from build123d import *

# Parameters (mm, degrees)
F0_W          = 25.4
F0_H          = 25.4
F1_DEPTH      = 584.2
F2_W          = 25.4
F2_H          = 25.4
F3_DEPTH      = 279.4
F3_DEPTH_BACK = 25.4
F5_DEPTH      = 584.201
F5_DEPTH_BACK = 584.201
F6_W          = 25.4
F6_H          = 25.4
F7_DEPTH      = 279.4
F8_W          = 25.4
F8_H          = 25.4
F9_DEPTH      = 355.6
F10_W         = 25.4
F10_H         = 25.4
F11_DEPTH     = 482.6
F12_R         = 3.96875
F13_DEPTH     = 1143.001
F14_W         = 25.4
F14_H         = 25.4
F15_DEPTH     = 152.4


with BuildPart() as f1:
    # F0 (on Right) → F1 (new body, symmetric)
    with BuildSketch(Plane.YZ):
        with Locations((12.7, 12.7)):
            Rectangle(F0_W, F0_H)
    extrude(amount=F1_DEPTH, both=True)



with BuildPart() as f1b:
    # F0 (on Right) → F1, piece 2 (new body, symmetric)
    with BuildSketch(Plane.YZ):
        with Locations((165.1, 12.7)):
            Rectangle(F0_W, F0_H)
    extrude(amount=F1_DEPTH, both=True)


with BuildPart() as f1_1:
    add(f1.part)

    add(f1b.part)  # F3 merges F1b
    # F2 (on Front) → F3 (join, two sides)
    with BuildSketch(Plane.XZ) as f3_sk:
        with Locations((-571.5, 12.7)):
            Rectangle(F2_W, F2_H)
        with Locations((-190.5, 12.7)):
            Rectangle(F2_W, F2_H)
        with Locations((63.5, 12.7)):
            Rectangle(F2_W, F2_H)
        with Locations((571.5, 12.7)):
            Rectangle(F2_W, F2_H)
    extrude(amount=-F3_DEPTH)
    extrude(f3_sk.sketch, amount=F3_DEPTH_BACK)

    # F4 (on Right) → F5 (cut, two sides)
    with BuildSketch(Plane.YZ) as f5_sk:
        with BuildLine():
            Line((215.9, 25.4), (244.475, 8.9022160579))
            ThreePointArc((244.475, 8.9022160579), (272.4008869908, 20.4694971908), (254, 44.45))
            Line((254, 44.45), (215.9, 44.45))
            Line((215.9, 44.45), (215.9, 25.4))
        make_face()
        Polygon((279.4, 4.0713296347), (279.4, 25.4), (273.685, 25.4), align=None)
    extrude(amount=F5_DEPTH, mode=Mode.SUBTRACT)
    extrude(f5_sk.sketch, amount=-F5_DEPTH_BACK, mode=Mode.SUBTRACT)

    # F6 (on Top) → F7 (join)
    with BuildSketch(Plane.XY):
        with Locations((-546.1, 190.5)):
            Rectangle(F6_W, F6_H)
        with Locations((-546.1, 139.7)):
            Rectangle(F6_W, F6_H)
        with Locations((-215.9, 139.7)):
            Rectangle(F6_W, F6_H)
        with Locations((-215.9, 190.5)):
            Rectangle(F6_W, F6_H)
        with Locations((88.9, 190.5)):
            Rectangle(F6_W, F6_H)
        with Locations((546.1, 190.5)):
            Rectangle(F6_W, F6_H)
        with Locations((546.1, 139.7)):
            Rectangle(F6_W, F6_H)
        with Locations((88.9, 139.7)):
            Rectangle(F6_W, F6_H)
    extrude(amount=F7_DEPTH)

    # F8 (on face) → F9 (join, through all)
    with BuildSketch(Plane(origin=(-558.8, 0, 0), x_dir=(0, -1, 0), z_dir=(-1, 0, 0))):
        with Locations((-165.1, 266.7)):
            Rectangle(F8_W, F8_H)
    extrude(amount=-F9_DEPTH)

    # F10 (on face) → F11 (join, through all)
    with BuildSketch(Plane.YZ.offset(558.8)):
        with Locations((165.1, 266.7)):
            Rectangle(F10_W, F10_H)
    extrude(amount=-F11_DEPTH)

    # F12 (on face) → F13 (cut, through all)
    with BuildSketch(Plane(origin=(-558.8, 0, 0), x_dir=(0, -1, 0), z_dir=(-1, 0, 0))):
        with Locations((-139.7, 101.6)):
            Circle(F12_R)
        with Locations((-139.7, 152.4)):
            Circle(F12_R)
        with Locations((-139.7, 203.2)):
            Circle(F12_R)
        with Locations((-139.7, 254)):
            Circle(F12_R)
        with Locations((-190.5, 101.6)):
            Circle(F12_R)
        with Locations((-190.5, 152.4)):
            Circle(F12_R)
        with Locations((-190.5, 203.2)):
            Circle(F12_R)
        with Locations((-190.5, 254)):
            Circle(F12_R)
    extrude(amount=-F13_DEPTH, mode=Mode.SUBTRACT)

    # F14 (on Top) → F15 (join)
    with BuildSketch(Plane.XY):
        with Locations((-546.1, -12.7)):
            Rectangle(F14_W, F14_H)
        with Locations((-215.9, -12.7)):
            Rectangle(F14_W, F14_H)
        with Locations((88.9, -12.7)):
            Rectangle(F14_W, F14_H)
        with Locations((546.1, -12.7)):
            Rectangle(F14_W, F14_H)
    extrude(amount=F15_DEPTH)


solid = f1_1.part
Work out the finished part from the listing and answer in its coordinate system (mm). A direction names the side the tool comes from. Round coordinates to 2 decimals unless told otherwise and drop trailing zeros. Write each loop counter-clockwise with the first axis right and the second up, starting at its lowest first coordinate (ties: lowest second). Pieces come first, ordered by that corner, then holes. Notation, with made-up numbers: (2, -22) - (23, -22) arc R27 cw to (23, -3) - close; hole circle Ø6 at (31.5, 31.5). An arc over 180 degrees is marked (long way). Answer in a Markdown table with one row per item. Add a question column.
1. A cutting plane is placed at B-B, the plane z = 169. Count the separate pieces of the cut face and the enclosed holes in it, and give its area (3 significant figures).
2. A cutting plane is placed at A-A, the plane x = 12. Determine the outline of the cut face in (y, z).
3. The mould has two halves that part along X. Classify faces 1 (the flat face through (-584.2, 129, 13)), 2 (the flat face through (558.8, 232, 10)), 3 (the flat face through (63.322, 229.987, 17.267)): +X half, -X half, draft (parallel to the pull), parting line (faces both ways), or undercut.
4. A cutting plane is placed at C-C, the plane x = 282. Determine the outline of the cut face in (y, z).
5. For faces 4 (the flat face through (-177.8, -13, 13)), 5 (the flat face through (533.4, 190, 138)), 6 (the flat face through (-546, 177.8, 138)), 7 (the flat face through (558.8, 181, 154)), determine the directions among +Z, -Z, +X, -X, +Y, -Y from which every point of the face is accessible in a straight line to the end or side of a thin tool.
6. Find the intervals of material crossed by line 1 along Y through (x, z) = (540, 203); line 2 along Z through (x, y) = (96, 139); line 3 along X through (y, z) = (198, 170.5), in increasing order. Write a range as from..to.
7. A cutting plane is placed at D-D, the plane y = 92. Determine the outline of the cut face in (x, z).
8. Given pin 1 (20.5 mm diameter, centred on x = 90.5, y = -8.5, fed in from +Z); pin 2 (7.5 mm diameter, centred on y = 186, z = 109.5, fed in from -X); pin 3 (12.5 mm diameter, centred on y = -11.5, z = 87, fed in from +X), each flat-ended and moving along its own axis, determine where each tip first touches the part or whether it passes through.
Worked out:
| question | item | result |
|---|---|---|
| 1 | separate pieces | 8 |
| 1 | enclosed holes | 0 |
| 1 | area | 5,160 mm^2 |
| 2 | outline | (0, 0) - (25.4, 0) - (25.4, 25.4) - (0, 25.4) - close; (152.4, 0) - (177.8, 0) - (177.8, 25.4) - (152.4, 25.4) - close |
| 3 | face 1 | -X half |
| 3 | face 2 | undercut |
| 3 | face 3 | draft |
| 4 | outline | (0, 0) - (25.4, 0) - (25.4, 25.4) - (0, 25.4) - close; (152.4, 0) - (177.8, 0) - (177.8, 25.4) - (152.4, 25.4) - close; (152.4, 254) - (177.8, 254) - (177.8, 279.4) - (152.4, 279.4) - close |
| 5 | face 4 | +Z, -Z, -Y |
| 5 | face 5 | +Z, -Z, +Y |
| 5 | face 6 | +X, -X |
| 5 | face 7 | +Z, +X, +Y, -Y |
| 6 | line 1 | 127..135.74, 143.66..152.4, 177.8..186.54, 194.46..203.2 |
| 6 | line 2 | 0..97.69, 105.51..148.49, 156.31..199.29, 207.11..250.09, 257.91..279.4 |
| 6 | line 3 | -558.8..-533.4, -228.6..-203.2, 76.2..101.6, 533.4..558.8 |
| 7 | outline | (-584.2, 0) - (-558.8, 0) - (-558.8, 25.4) - (-584.2, 25.4) - close; (-203.2, 0) - (-177.8, 0) - (-177.8, 25.4) - (-203.2, 25.4) - close; (50.8, 0) - (76.2, 0) - (76.2, 25.4) - (50.8, 25.4) - close; (558.8, 0) - (584.2, 0) - (584.2, 25.4) - (558.8, 25.4) - close |
| 8 | pin 1 | z = 152.4 |
| 8 | pin 2 | x = -558.8 |
| 8 | pin 3 | x = 558.8 |
